Autodesk Inventor part; units mm, degrees
ref_plane "YZ Plane" through (0, 0, 0) normal (1, 0, 0) x (0, 1, 0)
ref_plane "XZ Plane" through (0, 0, 0) normal (0, 1, 0) x (-1, 0, 0)
ref_plane "XY Plane" through (0, 0, 0) normal (0, 0, 1) x (1, 0, 0)
sketch "Skizze1" plane through (0, 0, 0) normal (0, 0, 1) x (1, 0, 0)
  circle A0 centre (0, 0) radius 13.7
  circle A1 centre (0, 0) radius 15
  dimension "d0" = 27.4
  dimension "d1" = 30
extrude "Extrusion1" add sketch "Skizze1" along normal blind 2
sketch "Skizze2" plane through (0, 0, 2) normal (0, 0, 1) x (1, 0, 0)
  circle A0 centre (0, 0) radius 15
  dimension "d4" = 30
extrude "Extrusion2" add sketch "Skizze2" along normal blind 9
sketch "Skizze3" plane through (0, 0, 2) normal (0, 0, -1) x (-1, 0, 0)
  circle A0 centre (3.25, 0) radius 2.1
  circle A1 centre (-3.25, 0) radius 3
  point P0 (0, 0)
  dimension "d7" = 4.2
  dimension "d8" = 6
  dimension "d10" = 3.25
  dimension "d11" = 3.25
  dimension "d12" = 6.5
extrude "Extrusion3" cut sketch "Skizze3" against normal blind 1.2
sketch "Skizze4" plane through (3.25, 0, 3.2) normal (0, 0, -1) x (-1, 0, 0)
  circle A0 centre (0, 0) radius 2.5
  circle A1 centre (6.5, 0) radius 2.1
  circle A2 centre (6.5, 0) radius 1.9
  point P0 (3.25, 0)
  dimension "d15" = 5
  dimension "d16" = 3.8
  dimension "d17" = 6.5
  dimension "d18" = 3.25
extrude "Extrusion4" cut sketch "Skizze4" against normal blind 3.4 contours A0 | A2
sketch "Skizze5" plane through (3.25, 0, 6.6) normal (0, 0, -1) x (-1, 0, 0)
  circle A0 centre (6.5, 0) radius 1.9
  circle A1 centre (6.5, 0) radius 1.6
  circle A2 centre (0, 0) radius 2.5
  point P0 (3.25, 0)
  dimension "d21" = 3.2
  dimension "d22" = 5
  dimension "d23" = 6.5
  dimension "d24" = 3.25
extrude "Extrusion5" cut sketch "Skizze5" against normal blind 4 contours A1 | A2
properties part number "schablone"
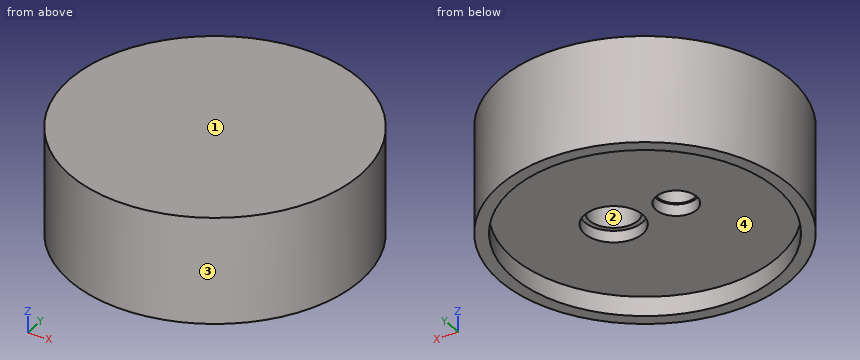
Could you check a few things on this model? Use its own coordinates, in mm. Face numbers are marked on the shaded views. Round coordinates to 2 decimals unless told otherwise and drop trailing zeros. Loops run counter-clockwise (first coordinate to the right, second up) from the corner with the lowest first, then second, coordinate; pieces in that order, holes last. Notation, with made-up numbers: (31, -12) - (82, -12) arc R20 cw to (82, 11) - close; hole circle Ø5 at (-7.75, -10). An arc over 180 degrees is marked (long way). Use CSV: the item, a comma, the result in double quotes.
Item 1: If we section it at C-C on x = -7: List the corners of the cut face in (y, z) for me.
Here are the results:
outline,"(-13.27, 0) - (-11.78, 0) - (-11.78, 2) - (11.78, 2) - (11.78, 0) - (13.27, 0) - (13.27, 11) - (-13.27, 11) - close"
Item 2: If we section it at B-B on z = 7.25: List the corners of the cut face in (x, y) for me, then the cut area to 3 significant figures.
Here are the results:
outline,"circle Ø30 at (0, 0); hole circle Ø3.2 at (-3.25, 0); hole circle Ø5 at (3.25, 0)"
area,"679 mm²"
Item 3: I need wall thicknesses on L1, parallel to Z at x = 7, y = -5; L2, parallel to Y at x = 3.25, z = 2.3; L3, parallel to Y at x = -3.25, z = 8.1. Which ranges of each line are inside material? Lowest first, please. Write a range as [from, to].
Here are the results:
L1,"z = [2, 11]"
L2,"y = [-14.64, -3], [3, 14.64]"
L3,"y = [-14.64, -1.6], [1.6, 14.64]"
Item 4: Will these pins go through, and if not, where does the flat tip stop? pin 1 (4 mm diameter, centred on x = -3.25, y = 0, fed in from -Z); pin 2 (1.8 mm diameter, centred on x = 4, y = 0.5, fed in from -Z); pin 3 (8 mm diameter, centred on x = 5.5, y = -2.5, fed in from -Z).
Here are the results:
pin 1,"stops at z = 3.2"
pin 2,"stops at z = 10.6"
pin 3,"stops at z = 2"
Item 5: If we section it at D-D on z = 1.5: List the corners of the cut face in (x, y) for me.
Here are the results:
outline,"circle Ø30 at (0, 0); hole circle Ø27.4 at (0, 0)"
Item 6: If we mould it in two halves opening along Y, with no side actions, what happens to the marked faces 1, 2, 3 and 4? For each: pulls with the +Y half, pulls with the -Y half, needs draft (parallel to the pull), parting line crosses it, or undercut.
Here are the results:
face 1,"needs draft"
face 2,"undercut"
face 3,"parting line crosses it"
face 4,"undercut"
Item 7: If we section it at A-A on y = 0: List the corners of the cut face in (x, z) for me.
Here are the results:
outline,"(-15, 0) - (-13.7, 0) - (-13.7, 2) - (-5.35, 2) - (-5.35, 3.2) - (-5.15, 3.2) - (-5.15, 6.6) - (-4.85, 6.6) - (-4.85, 10.6) - (-1.65, 10.6) - (-1.65, 6.6) - (-1.35, 6.6) - (-1.35, 3.2) - (-1.15, 3.2) - (-1.15, 2) - (0.25, 2) - (0.25, 3.2) - (0.75, 3.2) - (0.75, 10.6) - (5.75, 10.6) - (5.75, 3.2) - (6.25, 3.2) - (6.25, 2) - (13.7, 2) - (13.7, 0) - (15, 0) - (15, 11) - (-15, 11) - close"
